Part model, mm, in its own coordinate system. A direction names the side the tool comes from. Round coordinates to 2 decimals unless told otherwise and drop trailing zeros. Write each loop counter-clockwise with the first axis right and the second up, starting at its lowest first coordinate (ties: lowest second). Pieces come first, ordered by that corner, then holes.
1) Flat gauge pins, fed straight in: pin 1 (2 mm diameter, centred on x = 0, y = 0, fed in from +Z); pin 2 (2.5 mm diameter, centred on x = 0, y = 16, fed in from +Z); pin 3 (5 mm diameter, centred on x = 0.5, y = 8.5, fed in from +Z); pin 4 (5 mm diameter, centred on x = 13.5, z = 6, fed in from -Y). Where does each tip first touch, or does it go through?
2) Saw through at C-C on y = -16. Write the cut outline in (x, z).
3) Saw through at B-B on z = 3. Write the cut outline in (x, y), and give its area (3 significant figures).
4) Pull direction X, two halves, no side cores. Call faces 1 (the cylindrical face through (-16.75, -0.07, 14.49)), 2 (the flat face through (15, 0, 15.5)), 3 (the cylindrical face through (-2.343, -17.847, 0.986)): +X half, -X half, draft (parallel to the pull), parting line (faces both ways), or undercut.
5) Which spindle directions (+Z, -Z, +X, -X, +Y, -Y) get a long thin tool onto all of the face, cutting with end or side? Do faces 4 (the cylindrical face through (-16.837, 1.217, 7.67)), 5 (the flat face through (0, -16, 13.5)). Say none if no direction does.
6) Drill centre lines: L1, parallel to Y at x = 0, z = 1.5; L2, parallel to Z at x = -9, y = -3; L3, parallel to X at y = 1.5, z = 5.5. Where is each one in solid material? Low to high.
7) Saw through at D-D on x = -15.25. Write the cut outline in (y, z), and give its area (3 significant figures).
8) Saw through at A-A on x = 0. Write the cut outline in (y, z), and give its area (3 significant figures).
Autodesk Inventor part; units mm, degrees
ref_plane "YZ Plane" through (0, 0, 0) normal (1, 0, 0) x (0, 1, 0)
ref_plane "XZ Plane" through (0, 0, 0) normal (0, 1, 0) x (-1, 0, 0)
ref_plane "XY Plane" through (0, 0, 0) normal (0, 0, 1) x (1, 0, 0)
sketch "スケッチ1" plane through (0, 0, 0) normal (0, 0, 1) x (1, 0, 0)
  circle A0 centre (0, 0) radius 18
  dimension "d0" = 36
extrude "押し出し1" add sketch "スケッチ1" along normal blind 2
sketch "スケッチ2" plane through (0, 0, 2) normal (0, 0, 1) x (1, 0, 0)
  circle A0 centre (-15.25, 0) radius 2
  circle A1 centre (15.25, 0) radius 2
  point P0 (0, 0)
  dimension "d3" = 4
  dimension "d4" = 4
  dimension "d5" = 0
  dimension "d6" = 0
  dimension "d8" = 15.25
  dimension "d9" = 30.5
extrude "押し出し2" add sketch "スケッチ2" along normal blind 11.5
sketch "スケッチ3" plane through (-15.25, 0, 13.5) normal (0, 0, 1) x (1, 0, 0)
  circle A0 centre (0, 0) radius 1.5
  circle A1 centre (30.5, 0) radius 1.5
  circle A2 centre (0, 0) radius 2
  point P0 (15.25, 0)
  dimension "d12" = 3
  dimension "d13" = 3
  dimension "d14" = 30.5
  dimension "d15" = 0
extrude "押し出し3" add sketch "スケッチ3" along normal blind 2 contours A0 | A1
sketch "スケッチ4" plane through (0, 0, 2) normal (0, 0, 1) x (1, 0, 0)
  circle A0 centre (0, 16) radius 1.5
  circle A1 centre (0, -16) radius 1.5
  point P0 (0, 0)
  dimension "d18" = 3
  dimension "d19" = 3
  dimension "d20" = 32
  dimension "d21" = 16
extrude "押し出し4" add sketch "スケッチ4" along normal blind 11.5
sketch "スケッチ5" plane through (0, 0, 2) normal (0, 0, 1) x (1, 0, 0)
  circle A0 centre (0, 0) radius 1.4
  dimension "d24" = 2.8
extrude "押し出し5" cut sketch "スケッチ5" against normal blind 3
equation "\"BendRadius\" = Thickness"
equation "\"BendReliefWidth\" = Thickness"
equation "\"BendReliefDepth\" = 0.5 * Thickness"
equation "\"CornerReliefSize\" = 4 * Thickness"
equation "\"MinimumRemnant\" = 2 * Thickness"
equation "\"TransitionRadius\" = BendRadius"
equation "\"JacobiRadiusSize\" = BendRadius"
equation "\"GapSize\" = Thickness"
properties part number "1005"
Completed:
1. pin 1: passes through
1. pin 2: stops at z = 13.5
1. pin 3: stops at z = 2
1. pin 4: stops at y = -2
2. outline: (-8.25, 0) - (8.25, 0) - (8.25, 2) - (1.5, 2) - (1.5, 13.5) - (-1.5, 13.5) - (-1.5, 2) - (-8.25, 2) - close
3. outline: circle Ø4 at (-15.25, 0); circle Ø3 at (0, -16); circle Ø3 at (0, 16); circle Ø4 at (15.25, 0)
3. area: 39.3 mm2
4. face 1: undercut
4. face 2: draft
4. face 3: parting line
5. face 4: +Z
5. face 5: +Z, +X, -X, +Y, -Y
6. L1: y = -18 to -1.4, 1.4 to 18
6. L2: z = 0 to 2
6. L3: x = -16.57 to -13.93, 13.93 to 16.57
7. outline: (-9.56, 0) - (9.56, 0) - (9.56, 2) - (2, 2) - (2, 13.5) - (1.5, 13.5) - (1.5, 15.5) - (-1.5, 15.5) - (-1.5, 13.5) - (-2, 13.5) - (-2, 2) - (-9.56, 2) - close
7. area: 90.2 mm2
8. outline: (-18, 0) - (-1.4, 0) - (-1.4, 2) - (-14.5, 2) - (-14.5, 13.5) - (-17.5, 13.5) - (-17.5, 2) - (-18, 2) - close; (1.4, 0) - (18, 0) - (18, 2) - (17.5, 2) - (17.5, 13.5) - (14.5, 13.5) - (14.5, 2) - (1.4, 2) - close
8. area: 135 mm2
